from build123d import *

# Parameters (mm, degrees)
SKETCH_1_W          = 30
SKETCH_1_H          = 25
SKETCH_1_R          = 1.5
SKETCH_1_R_2        = 4
EXTRUDE_1_DEPTH     = 4
SKETCH_2_W          = 4
SKETCH_2_H          = 25
EXTRUDE_2_DEPTH     = 80
SKETCH_3_W          = 30
SKETCH_3_H          = 25
EXTRUDE_3_DEPTH     = 4
CUT_EXTRUDE_START   = -11
SKETCH_4_R          = 1.5
SKETCH_4_R_2        = 4
CUT_EXTRUDE_1_DEPTH = 11
EXTRUDE_4_DEPTH     = 25


with BuildPart() as part:
    # 草图1 → 凸台-拉伸1 (new body)
    with BuildSketch(Plane.XY):
        Rectangle(SKETCH_1_W, SKETCH_1_H)
        with Locations((7, 0)):
            Circle(SKETCH_1_R, mode=Mode.SUBTRACT)
        with Locations((0, 7)):
            Circle(SKETCH_1_R, mode=Mode.SUBTRACT)
        with Locations((-7, 0)):
            Circle(SKETCH_1_R, mode=Mode.SUBTRACT)
        with Locations((0, -7)):
            Circle(SKETCH_1_R, mode=Mode.SUBTRACT)
        Circle(SKETCH_1_R_2, mode=Mode.SUBTRACT)
    extrude(amount=EXTRUDE_1_DEPTH)

    # 草图2 → 凸台-拉伸2 (add)
    with BuildSketch(Plane.XY.offset(4)):
        with Locations((-13, 0)):
            Rectangle(SKETCH_2_W, SKETCH_2_H)
        with Locations((13, 0)):
            Rectangle(SKETCH_2_W, SKETCH_2_H)
    extrude(amount=EXTRUDE_2_DEPTH)

    # 草图3 → 凸台-拉伸3 (add)
    with BuildSketch(Plane.XY.offset(84)):
        Rectangle(SKETCH_3_W, SKETCH_3_H)
    extrude(amount=EXTRUDE_3_DEPTH)

    # 草图4 → 切除-拉伸1 (cut)
    with BuildSketch(Plane.XY.offset(88).offset(CUT_EXTRUDE_START)):
        with Locations((-7, 0)):
            Circle(SKETCH_4_R)
        with Locations((0, -7)):
            Circle(SKETCH_4_R)
        with Locations((7, 0)):
            Circle(SKETCH_4_R)
        Circle(SKETCH_4_R_2)
        with Locations((0, 7)):
            Circle(SKETCH_4_R)
    extrude(amount=CUT_EXTRUDE_1_DEPTH, mode=Mode.SUBTRACT)

    # 草图9 → 凸台-拉伸4 (add)
    with BuildSketch(Plane.XZ.offset(12.5)):
        Polygon((11, 58.385569275), (-11, 70.493433903), (-11, 65.927659735), (6.349452589, 56.379258675), align=None)
        Polygon((11, 53.819795107), (11, 58.385569275), (6.349452589, 56.379258675), align=None)
        Polygon((-6.349452589, 46.335000836), (11, 53.819795107), (6.349452589, 56.379258675), (-11, 48.894464404), align=None)
        Polygon((-6.349452589, 46.335000836), (-11, 48.894464404), (-11, 44.328690237), align=None)
        Polygon((11, 36.786599776), (-6.349452589, 46.335000836), (-11, 44.328690237), (6.349452589, 34.780289177), align=None)
        Polygon((11, 32.220825609), (11, 36.786599776), (6.349452589, 34.780289177), align=None)
        Polygon((-11, 22.729720739), (11, 32.220825609), (6.349452589, 34.780289177), (-11, 27.295494906), align=None)
    extrude(amount=-EXTRUDE_4_DEPTH)


solid = part.part
Input: part model. Units: mm. Frame: model coordinates. A direction names the side the tool comes from. Round coordinates to 2 decimals unless told otherwise and drop trailing zeros. Order: outer loops, then holes, each group sorted by start corner. A loop starts at its lowest first (then second) coordinate and runs counter-clockwise, first axis right, second up.
1. Cut plane A-A, the plane z = 77.5. Output: boundary loops of the cut face in (x, y).
The answers:
outline: (-15, -12.5) - (-11, -12.5) - (-11, 12.5) - (-15, 12.5) - close; (11, -12.5) - (15, -12.5) - (15, 12.5) - (11, 12.5) - close
2. Cut plane C-C, the plane x = -9.75. Output: boundary loops of the cut face in (y, z), then the cut area to 3 significant figures.
The answers:
outline: (-12.5, 0) - (12.5, 0) - (12.5, 4) - (-12.5, 4) - close; (-12.5, 23.27) - (12.5, 23.27) - (12.5, 27.83) - (-12.5, 27.83) - close; (-12.5, 43.64) - (12.5, 43.64) - (12.5, 49.43) - (-12.5, 49.43) - close; (-12.5, 65.24) - (12.5, 65.24) - (12.5, 69.81) - (-12.5, 69.81) - close; (-12.5, 84) - (12.5, 84) - (12.5, 88) - (-12.5, 88) - close
area: 573 mm2
3. Material intervals for line 1 (X direction, y = 0, z = 85.25); line 2 (Y direction, x = 0, z = 3.2); line 3 (X direction, y = -2.75, z = 65), sorted ascending.
The answers:
line 1: x = -15 to -8.5, -5.5 to -4, 4 to 5.5, 8.5 to 15
line 2: y = -12.5 to -8.5, -5.5 to -4, 4 to 5.5, 8.5 to 12.5
line 3: x = -15 to -11, -9.31 to -1.02, 11 to 15
4. Cut plane B-B, the plane y = 10.25. Output: boundary loops of the cut face in (x, z) (1 decimal).
The answers:
outline: (-15, 0) - (15, 0) - (15, 88) - (-15, 88) - close; hole (-11, 4) - (11, 4) - (11, 32.2) - (-11, 22.7) - close; hole (-11, 27.3) - (6.3, 34.8) - (-11, 44.3) - close; hole (-11, 48.9) - (6.3, 56.4) - (-11, 65.9) - close; hole (-11, 70.5) - (11, 58.4) - (11, 84) - (-11, 84) - close; hole (-6.3, 46.3) - (11, 36.8) - (11, 53.8) - close
5. Mould query, pull axis X, two halves, no side actions, for faces 4 (the face through (-2.2, -0.18, 31.09)), 5 (the face through (-4, 3, 0)), 6 (the face through (15, 0, 43)). Classes: released by +X, released by -X, zero draft, split by the parting line, or undercut.
The answers:
face 4: undercut
face 5: zero draft
face 6: released by +X
6. Pin query (flat end, axial travel): P1, Ø7, axis at x = 0, y = 0, coming from the -Z side; P2, Ø5, axis at x = 0, y = -7, coming from the -Z side; P3, Ø2, axis at x = 0, y = 7, coming from the +Z side; P4, Ø1.8, axis at x = 0, y = 7, coming from the +Z side. Return the tip coordinate at first contact, or that it passes through.
The answers:
P1: stops at z = 25.97
P2: stops at z = 0
P3: stops at z = 64.99
P4: stops at z = 64.93
7. Set-up query: faces 1 (the face through (-0.325, -8.464, 1.972)), 2 (the face through (-0.325, -8.464, 85.972)), 3 (the face through (-2.45, -0.18, 61.22)). Return all of +Z, -Z, +X, -X, +Y, -Y with unobstructed straight access to the full face (end or side cutting, diameter ignored); none if empty.
The answers:
face 1: -Z
face 2: +Z
face 3: +Y, -Y
8. Cut plane D-D, the plane y = 2.75. State how many separate pieces and enclosed holes the cut face has, then the cut area to 3 significant figures.
The answers:
separate pieces: 1
enclosed holes: 3
area: 1,200 mm2
